The listing builds one solid part. Answer for the finished solid, in the listing's coordinates (mm). A direction names the side the tool comes from. Give positions to 0.01 mm unless a question says otherwise; leave off trailing zeros. Order: outer loops, then holes, each group sorted by start corner. A loop starts at its lowest first (then second) coordinate and runs counter-clockwise, first axis right, second up. Notation, with made-up numbers: (67.25, 37) - (103.25, 37) arc R24 cw to (103.25, 57) - close; hole circle Ø8 at (22.5, 57.25). An arc over 180 degrees is marked (long way). Answer as a JSON object with one key per item and string values. Group by question number.
Q1. A cutting plane is placed at B-B, the plane z = 90. Give the vertices of the cut face in (x, y).
Q2. A cutting plane is placed at A-A, the plane x = 70. Give the vertices of the cut face in (y, z), and give its area (3 significant figures).
Q3. Given pin 1 (2.5 mm diameter, centred on x = 8, y = 3, fed in from -Z); pin 2 (1.6 mm diameter, centred on x = -3, y = 2, fed in from -Z); pin 3 (1.6 mm diameter, centred on y = 3, z = 2, fed in from +X), each flat-ended and moving along its own axis, determine where each tip first touches the part or whether it passes through.
Q4. A cutting plane is placed at D-D, the plane y = 3. Give the vertices of the cut face in (x, z).
Q5. A cutting plane is placed at C-C, the plane x = 8.5. Give the vertices of the cut face in (y, z).
Q6. For faces 1 (the face through (110, 3, 3)), 2 (the face through (15, 3, 5.2)), 3 (the face through (55, 3, 3)), determine the directions among +Z, -Z, +X, -X, +Y, -Y from which every point of the face is accessible in a straight line to the end or side of a thin tool.
Q7. The mould has two halves that part along X. Classify faces 4 (the face through (85, 3, 3)), 5 (the face through (-3, 3, 15)), 6 (the face through (30, 3, 3)): released by +X, released by -X, zero draft, split by the parting line, or undercut.
Q8. Consider line 1 (Z direction, x = 8.5, y = 1.9); line 2 (Z direction, x = 39.5, y = 2.2); line 3 (Z direction, x = 70, y = 3.45). Determine where each line is inside the solid, lowest interval first.
Autodesk Inventor part; units mm, degrees
ref_plane "YZ Plane" through (0, 0, 0) normal (1, 0, 0) x (0, 1, 0)
ref_plane "XZ Plane" through (0, 0, 0) normal (0, 1, 0) x (-1, 0, 0)
ref_plane "XY Plane" through (0, 0, 0) normal (0, 0, 1) x (1, 0, 0)
sketch "Sketch1" plane through (0, 0, 0) normal (0, 1, 0) x (-1, 0, 0)
  line L0 (0, 0) -> (-140, 0)
  line L1 (-140, 0) -> (-140, 60)
  line L2 (-78.4315, 105) -> (-61.5685, 105)
  line L3 (0, 60) -> (-33.2843, 93.2843)
  line L4 (-140, 60) -> (-106.7157, 93.2843)
  arc A0 (-33.2843, 93.2843) -> (-61.5685, 105) centre (-61.5685, 65) ccw
  arc A1 (-78.4315, 105) -> (-106.7157, 93.2843) centre (-78.4315, 65) ccw
  circle A2 centre (-70, 90) radius 2.5
  line L5 (-85, 0) -> (-85, 5.2)
  line L6 (-85, 5.2) -> (-55, 5.2)
  line L7 (-55, 5.2) -> (-55, 0)
  circle A3 centre (-24, 30.7632) radius 11.5
  circle A4 centre (-39.5, 46.2632) radius 1.5
  circle A5 centre (-39.5, 15.2632) radius 1.5
  circle A6 centre (-8.5, 15.2632) radius 1.5
  circle A7 centre (-8.5, 46.2632) radius 1.5
  line L8 (-30, 0) -> (0, 0)
  line L9 (0, 0) -> (0, 5.2)
  line L10 (0, 5.2) -> (-30, 5.2)
  line L11 (-30, 5.2) -> (-30, 0)
  line L12 (-110, 0) -> (-140, 0)
  line L13 (-140, 0) -> (-140, 5.2)
  line L14 (-140, 5.2) -> (-110, 5.2)
  line L15 (-110, 5.2) -> (-110, 0)
  line L16 (0, 45) -> (5.2, 45)
  line L17 (5.2, 45) -> (5.2, 15)
  line L18 (5.2, 15) -> (0, 15)
  line L19 (0, 60) -> (0, 45)
  line L20 (0, 15) -> (0, 0)
  point P0 (-45, 105)
  point P1 (-95, 105)
  point P2 (-70, 105)
  dimension "d0" = 140
  dimension "d1" = 60
  dimension "d3" = 135
  dimension "d4" = 50
  dimension "d5" = 40
  dimension "d8" = 5
  dimension "d12" = 90
  dimension "d13" = 30
  dimension "d14" = 15
  dimension "d15" = 5.2
  dimension "d16" = 23
  dimension "d17" = 75
  dimension "d18" = 3
  dimension "d19" = 15.5
  dimension "d20" = 15.5
  dimension "d23" = 360
  dimension "d25" = 30
  dimension "d26" = 5.2
  dimension "d28" = 30
  dimension "d29" = 5.2
  dimension "d35" = 30
  dimension "d36" = 15
  dimension "d37" = 24
  dimension "d38" = 15
  dimension "d39" = 5.2
  dimension "d40" = 5.2
  dimension "d41" = 70
extrude "Extrusion3" add sketch "Sketch1" along normal blind 5.2 contours L0 L7 L6 L5 L15 L14 L1 L4 A1 L2 A0 L3 L19 L16 L17 L18 L20 L10 L11
properties part number "side Plate"
Reply:
{
 "1": {"outline": "(30, 0) - (67.5, 0) - (67.5, 5.2) - (30, 5.2) - close; (72.5, 0) - (110, 0) - (110, 5.2) - (72.5, 5.2) - close"},
 "2": {"outline": "(0, 5.2) - (5.2, 5.2) - (5.2, 87.5) - (0, 87.5) - close; (0, 92.5) - (5.2, 92.5) - (5.2, 105) - (0, 105) - close", "area": "493 mm^2"},
 "3": {"pin 1": "stops at z = 5.2", "pin 2": "stops at z = 15", "pin 3": "stops at x = 110"},
 "4": {"outline": "(-5.2, 15) - (0, 15) - (0, 5.2) - (30, 5.2) - (30, 0) - (55, 0) - (55, 5.2) - (85, 5.2) - (85, 0) - (110, 0) - (110, 5.2) - (140, 5.2) - (140, 60) - (106.72, 93.28) arc R40 ccw to (78.43, 105) - (61.57, 105) arc R40 ccw to (33.28, 93.28) - (0, 60) - (0, 45) - (-5.2, 45) - close; hole circle Ø3 at (8.5, 15.26); hole circle Ø3 at (8.5, 46.26); hole circle Ø23 at (24, 30.76); hole circle Ø3 at (39.5, 15.26); hole circle Ø3 at (39.5, 46.26); hole circle Ø5 at (70, 90)"},
 "5": {"outline": "(0, 5.2) - (5.2, 5.2) - (5.2, 13.76) - (0, 13.76) - close; (0, 16.76) - (5.2, 16.76) - (5.2, 44.76) - (0, 44.76) - close; (0, 47.76) - (5.2, 47.76) - (5.2, 68.5) - (0, 68.5) - close"},
 "6": {"face 1": "-Z, +X, +Y, -Y", "face 2": "-Z, -X, +Y, -Y", "face 3": "-Z, +Y, -Y"},
 "7": {"face 4": "undercut", "face 5": "zero draft", "face 6": "released by -X"},
 "8": {"line 1": "z = 5.2 to 13.76, 16.76 to 44.76, 47.76 to 68.5", "line 2": "z = 0 to 13.76, 16.76 to 44.76, 47.76 to 98.36", "line 3": "z = 5.2 to 87.5, 92.5 to 105"}
}
